```python
from build123d import *

# Parameters (mm, degrees)
EXTRUDE_1_DEPTH     = 15
SKETCH_2_R          = 1.45
CUT_EXTRUDE_1_DEPTH = 29.071464012
SKETCH_3_R          = 1.65
CUT_EXTRUDE_2_DEPTH = 29.071464012


with BuildPart() as part:
    # 草图1 → 凸台-拉伸1 (new body)
    with BuildSketch(Plane(origin=(0, 0, 0), x_dir=(1, 0, 0), z_dir=(0, 1, 0))):
        Polygon((0, 0), (0, -10), (19.947198592, -11.452332033), (20.781029397, 0), align=None)
    extrude(amount=EXTRUDE_1_DEPTH)

    # 草图2 → 切除-拉伸1 (cut, through all)
    with BuildSketch(Plane.XZ):
        with Locations(Location((5, 5, 0), (0, 0, 270))):
            Circle(SKETCH_2_R)
        with Locations(Location((15, 5, 0), (0, 0, 270))):
            Circle(SKETCH_2_R)
    extrude(amount=-CUT_EXTRUDE_1_DEPTH, mode=Mode.SUBTRACT)

    # 草图3 → 切除-拉伸2 (cut, through all)
    with BuildSketch(Plane.XZ):
        with Locations(Location((5, 5, 0), (0, 0, 270))):
            Circle(SKETCH_3_R)
        with Locations(Location((15, 5, 0), (0, 0, 270))):
            Circle(SKETCH_3_R)
    extrude(amount=-CUT_EXTRUDE_2_DEPTH, mode=Mode.SUBTRACT)


solid = part.part
```
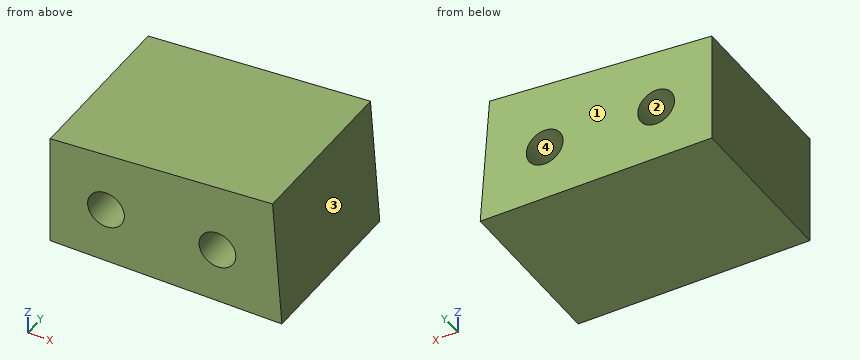
Can you work these out from the model? Positions are in its coordinate system, mm. Face numbers are marked on the shaded views. Coordinates: 2 decimals unless noted, no trailing zeros. Order: outer loops, then holes, each group sorted by start corner. A loop starts at its lowest first (then second) coordinate and runs counter-clockwise, first axis right, second up. Notation, with made-up numbers: (64, 31) - (92, 31) arc R12 cw to (92, 46) - close; hole circle Ø6 at (13.5, 28.5). An arc over 180 degrees is marked (long way). Answer in a Markdown table with one row per item.
1. Suppose I cut it at D-D (x = 6). Please give me the cut outline in (y, z), and give its area (3 significant figures).
Reply:
| item | result |
|---|---|
| outline | (0, 0) - (15, 0) - (15, 3.69) - (0, 3.69) - close; (0, 6.31) - (15, 6.31) - (15, 10.44) - (0, 10.44) - close |
| area | 117 mm^2 |
2. Suppose I cut it at A-A (x = 15). Please give me the cut outline in (y, z), and give its area (3 significant figures).
Reply:
| item | result |
|---|---|
| outline | (0, 0) - (15, 0) - (15, 3.35) - (0, 3.35) - close; (0, 6.65) - (15, 6.65) - (15, 11.09) - (0, 11.09) - close |
| area | 117 mm^2 |
3. If I drill on line 1 along X through (y, z) = (4, 5); line 2 along X through (y, z) = (3.5, 3.75); line 3 along Z through (x, y) = (16.5, 2.75), over which ranges is the centre line in solid material (lowest first)?
Reply:
| item | result |
|---|---|
| line 1 | x = 0 to 3.35, 6.65 to 13.35, 16.65 to 20.42 |
| line 2 | x = 0 to 3.92, 6.08 to 13.92, 16.08 to 20.51 |
| line 3 | z = 0 to 4.31, 5.69 to 11.2 |
4. If we mould it in two halves opening along Z, with no side actions, what happens to the marked faces 1, 2, 3 and 4? For each: pulls with the +Z half, pulls with the -Z half, needs draft (parallel to the pull), parting line crosses it, or undercut.
Reply:
| item | result |
|---|---|
| face 1 | needs draft |
| face 2 | undercut |
| face 3 | pulls with the +Z half |
| face 4 | undercut |
5. Suppose I cut it at B-B (z = 5). Please give me the cut outline in (x, y), and give its area (3 significant figures).
Reply:
| item | result |
|---|---|
| outline | (0, 0) - (3.35, 0) - (3.35, 15) - (0, 15) - close; (6.65, 0) - (13.35, 0) - (13.35, 15) - (6.65, 15) - close; (16.65, 0) - (20.42, 0) - (20.42, 15) - (16.65, 15) - close |
| area | 207 mm^2 |
6. Suppose I cut it at C-C (y = 12). Please give me the cut outline in (x, z).
Reply:
| item | result |
|---|---|
| outline | (0, 0) - (20.78, 0) - (19.95, 11.45) - (0, 10) - close; hole circle Ø3.3 at (5, 5); hole circle Ø3.3 at (15, 5) |
7. For pin 1 (2 mm diameter, centred on x = 13.5, y = 4.5, fed in from +Z); pin 2 (3 mm diameter, centred on x = 5, z = 5, fed in from +Y), each with a flat end and sliding along its axis, tell me the tip position at first contact or that it passes through.
Reply:
| item | result |
|---|---|
| pin 1 | stops at z = 11.06 |
| pin 2 | passes through |
